Here's how the part is built. I have some questions about the finished solid (model axes, mm). Round coordinates to 2 decimals unless told otherwise and drop trailing zeros. Order: outer loops, then holes, each group sorted by start corner. A loop starts at its lowest first (then second) coordinate and runs counter-clockwise, first axis right, second up. Notation, with made-up numbers: (80, 3.25) - (89, 3.25) arc R12 ccw to (89, 17.25) - close; hole circle Ø5 at (43.5, 4.25). An arc over 180 degrees is marked (long way). One line per item, written item: value.
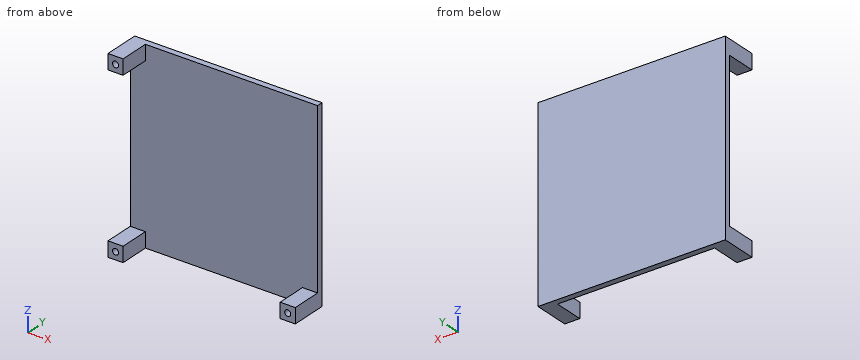
from build123d import *

# Parameters (mm, degrees)
SKETCH2_W           = 62
SKETCH2_H           = 62
BOSS_EXTRUDE1_DEPTH = 2
SKETCH3_W           = 5
SKETCH3_H           = 5
BOSS_EXTRUDE2_DEPTH = 10
SKETCH6_R           = 1
CUT_EXTRUDE2_DEPTH  = 3
CIRPATTERN1_COUNT   = 3
CIRPATTERN1_ANGLE   = 180


with BuildPart() as part:
    # Sketch2 → Boss-Extrude1 (new body)
    with BuildSketch(Plane(origin=(0, 0, 0), x_dir=(1, 0, 0), z_dir=(0, 1, 0))):
        Rectangle(SKETCH2_W, SKETCH2_H)
    extrude(amount=BOSS_EXTRUDE1_DEPTH)

    # Sketch3 → Boss-Extrude2 (add)
    with BuildSketch(Plane.XZ):
        with Locations((-28.5, 28.5)):
            Rectangle(SKETCH3_W, SKETCH3_H)
    boss_extrude2 = extrude(amount=BOSS_EXTRUDE2_DEPTH)

    # Sketch6 → Cut-Extrude2 (cut)
    with BuildSketch(Plane.XZ.offset(10)):
        with Locations((-28.5, 28.5)):
            Circle(SKETCH6_R)
    cut_extrude2 = extrude(amount=-CUT_EXTRUDE2_DEPTH, mode=Mode.SUBTRACT)

    # CirPattern1: Boss-Extrude2, Cut-Extrude2 ×3 about axis
    cirpattern1_axis = Axis((0, 0, 0), (0, -1, 0))
    for i in range(1, CIRPATTERN1_COUNT):
        add(boss_extrude2.rotate(cirpattern1_axis, i * CIRPATTERN1_ANGLE / (CIRPATTERN1_COUNT - 1)))
        add(cut_extrude2.rotate(cirpattern1_axis, i * CIRPATTERN1_ANGLE / (CIRPATTERN1_COUNT - 1)), mode=Mode.SUBTRACT)


solid = part.part
Q1. If we section it at C-C, the plane z = -28.5: Please give me the cut outline in (x, y).
Results list:
outline: (-31, -10) - (-29.5, -10) - (-29.5, -7) - (-27.5, -7) - (-27.5, -10) - (-26, -10) - (-26, 0) - (26, 0) - (26, -10) - (27.5, -10) - (27.5, -7) - (29.5, -7) - (29.5, -10) - (31, -10) - (31, 2) - (-31, 2) - close
Q2. If we section it at D-D, the plane x = 28.5: Please give me the cut outline in (y, z), then the cut area to 3 significant figures.
Results list:
outline: (-10, -31) - (2, -31) - (2, 31) - (0, 31) - (0, -26) - (-10, -26) - (-10, -27.5) - (-7, -27.5) - (-7, -29.5) - (-10, -29.5) - close
area: 168 mm²
Q3. Will these pins go through, and if not, where does the flat tip stop? pin 1 (5.5 mm diameter, centred on x = 28.5, y = -5, fed in from +Z); pin 2 (1.5 mm diameter, centred on x = -10, z = -21, fed in from -Y); pin 3 (0.6 mm diameter, centred on x = -28.5, z = 28, fed in from -Y).
Results list:
pin 1: z = -26
pin 2: y = 0
pin 3: y = -7
Q4. If we section it at B-B, the plane y = -8.5: Please give me the cut outline in (x, z).
Results list:
outline: (-31, -31) - (-26, -31) - (-26, -26) - (-31, -26) - close; (-31, 26) - (-26, 26) - (-26, 31) - (-31, 31) - close; (26, -31) - (31, -31) - (31, -26) - (26, -26) - close; hole circle Ø2 at (-28.5, -28.5); hole circle Ø2 at (-28.5, 28.5); hole circle Ø2 at (28.5, -28.5)
Q5. If I drill on line 1 along Z through (x, y) = (-28.5, -7.85); line 2 along Y through (x, z) = (6, 19), over which ranges is the centre line in solid material (lowest first)?
Results list:
line 1: -31 to -29.5, -27.5 to -26, 26 to 27.5, 29.5 to 31
line 2: 0 to 2
Q6. If we section it at A-A, the plane y = -2.5: Please give me the cut outline in (x, z), then the cut area to 3 significant figures.
Results list:
outline: (-31, -31) - (-26, -31) - (-26, -26) - (-31, -26) - close; (-31, 26) - (-26, 26) - (-26, 31) - (-31, 31) - close; (26, -31) - (31, -31) - (31, -26) - (26, -26) - close
area: 75.0 mm²
